```python
from build123d import *

# Parameters (mm, degrees)
F0_W        = 53.975
F0_H        = 76.2
F1_DEPTH    = 3.175
F2_W        = 47.625
F2_H        = 69.85
F3_DEPTH    = 5.08
F4_T        = 3.175
F4_T3_DEPTH = 53.975
F4_T5_DEPTH = 76.2
F5_W        = 25.4
F5_H        = 38.1
F6_DEPTH    = 25.4


# Not quite as in the source:
# - a shell that OpenCascade refuses in one call is made with other operations: the cavity is built on its own and cut out


with BuildPart() as f1:
    # F0 (on Top) → F1 (new body)
    with BuildSketch(Plane.XY):
        Rectangle(F0_W, F0_H)
    extrude(amount=F1_DEPTH)

    # F2 (on face) → F3 (join)
    with BuildSketch(Plane.XY.offset(3.175)):
        Rectangle(F2_W, F2_H)
    extrude(amount=F3_DEPTH)

    # F4: shell of thickness 3.175, made by hand


with BuildPart() as f4_core1:
    # F4_t2: copy of F1
    add(f1.part)

    # the walls: a layer under each face that stays
    f4_faces = [f4_core1.faces().sort_by_distance(p)[0] for p in [
        (0, 38.1, 1.5875),
        (26.9875, 0, 1.5875),
        (-26.9875, 0, 1.5875),
        (0, 0, 0),
        (-25.1883333333, -35.56, 3.175),
        (0, -38.1, 1.5875),
        (0, 34.925, 5.715),
        (-23.8125, 0, 5.715),
        (0, -34.925, 5.715),
        (23.8125, 0, 5.715),
    ]]
    thicken(f4_faces, amount=-F4_T, mode=Mode.SUBTRACT)

    # F4_s4 → F4_t3 (cut)
    with BuildSketch(Plane.YZ.offset(-26.9875)):
        Polygon((34.95675, 3.20675), (34.925, 0), (31.75, 0), (31.75, 3.175), align=None)
        Polygon((-34.95675, 3.20675), (-34.925, 0), (-31.75, 0), (-31.75, 3.175), align=None)
    extrude(amount=F4_T3_DEPTH, mode=Mode.SUBTRACT)

    # F4_s6 → F4_t5 (cut)
    with BuildSketch(Plane.XZ.offset(-38.1)):
        Polygon((-23.84425, 3.20675), (-23.8125, 0), (-20.6375, 0), (-20.6375, 3.175), align=None)
        Polygon((23.84425, 3.20675), (23.8125, 0), (20.6375, 0), (20.6375, 3.175), align=None)
    extrude(amount=F4_T5_DEPTH, mode=Mode.SUBTRACT)


with BuildPart() as f1_1:
    add(f1.part)

    # what is left inside the walls is the cavity
    f4_cavity = [f4_core1.part.solids().sort_by_distance(p)[0] for p in [
        (0, -10.583333, 3.20675),
    ]]
    add(f4_cavity, mode=Mode.SUBTRACT)

    # F5 (on face) → F6 (cut)
    with BuildSketch(Plane.XY.offset(3.175)):
        Rectangle(F5_W, F5_H)
    extrude(amount=-F6_DEPTH, mode=Mode.SUBTRACT)


solid = f1_1.part
```
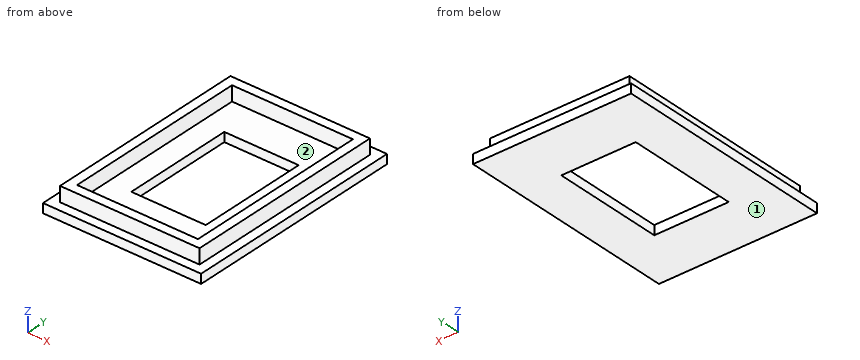
Part model, mm, in its own coordinate system. Face numbers are marked on the shaded views. Round coordinates to 2 decimals unless told otherwise and drop trailing zeros. Order: outer loops, then holes, each group sorted by start corner. A loop starts at its lowest first (then second) coordinate and runs counter-clockwise, first axis right, second up. Notation, with made-up numbers: M 36.25,57 L 87.25,57 A9 cw 87.25,61 Z; hole C 14.5,70.25 d1. An arc over 180 degrees is marked long. Put each result on its own line as item: value. Start each with the question number.
1. Drill centre lines: probe 1 along Y at (x, z) = (-15, 6.5) (3 decimals); probe 2 along X at (y, z) = (-30, 7); probe 3 along X at (y, z) = (10, 1.5). Where is each one in solid material? Low to high. Write a range as [from, to].
2. Slice it at D-D on x = -22. List the corners of the cut face in (y, z) (3 decimals), then the cut area to 3 significant figures.
3. Two-plate mould, pull along X, no slides. Class the marked faces 1 and 2: +X half, -X half, draft (parallel to the pull), parting line (faces both ways), or undercut.
4. Slice it at B-B on y = -14.5. List the corners of the cut face in (x, z) (1 decimal).
5. Slice it at C-C on x = 7. List the corners of the cut face in (y, z) (3 decimals), then the cut area to 3 significant figures.
6. Drop flat-ended pins along their axis: pin 1 (2.5 mm diameter, centred on x = 7.5, z = 6, fed in from -Y) (3 decimals); pin 2 (4 mm diameter, centred on y = -5, z = 6, fed in from +X); pin 3 (5 mm diameter, centred on x = -5.5, y = 24.5, fed in from +Z) (3 decimals). Give the stop position or say it passes through.
Findings:
1. probe 1: [-34.925, -31.75], [31.75, 34.925]
1. probe 2: [-23.81, -20.64], [20.64, 23.81]
1. probe 3: [-26.99, -12.7], [12.7, 26.99]
2. outline: M -38.1,0 L 38.1,0 L 38.1,3.175 L 34.925,3.175 L 34.925,8.255 L -34.925,8.255 L -34.925,3.175 L -38.1,3.175 Z
2. area: 597 mm2
3. face 1: draft
3. face 2: undercut
4. outline: M -27,0 L -12.7,0 L -12.7,3.2 L -20.6,3.2 L -20.6,8.3 L -23.8,8.3 L -23.8,3.2 L -27,3.2 Z; M 12.7,0 L 27,0 L 27,3.2 L 23.8,3.2 L 23.8,8.3 L 20.6,8.3 L 20.6,3.2 L 12.7,3.2 Z
5. outline: M -38.1,0 L -19.05,0 L -19.05,3.175 L -31.75,3.175 L -31.75,8.255 L -34.925,8.255 L -34.925,3.175 L -38.1,3.175 Z; M 19.05,0 L 38.1,0 L 38.1,3.175 L 34.925,3.175 L 34.925,8.255 L 31.75,8.255 L 31.75,3.175 L 19.05,3.175 Z
5. area: 153 mm2
6. pin 1: y = -34.925
6. pin 2: x = 23.81
6. pin 3: z = 3.175
